Can you work these out from the model? Positions are in its coordinate system, mm. A direction names the side the tool comes from. Give positions to 0.01 mm unless a question says otherwise; leave off trailing zeros. Order: outer loops, then holes, each group sorted by start corner. A loop starts at its lowest first (then second) coordinate and runs counter-clockwise, first axis right, second up. Notation, with made-up numbers: M -15,33 L 40,33 A35 cw 40,70 Z; hole C 68.25,47 d5. An arc over 180 degrees is marked long. Write each question's results on one line, items separated by ' | '.
from build123d import *

# Parameters (mm, degrees)
SKETCH_1_R      = 1.5
SKETCH_1_W      = 87
SKETCH_1_H      = 57
EXTRUDE_2_DEPTH = 3
SKETCH_3_W      = 3
SKETCH_3_H      = 67
EXTRUDE_3_DEPTH = 2


with BuildPart() as part:
    # 草图1 → 凸台-拉伸2 (new body)
    with BuildSketch(Plane.XY):
        Polygon((-11.864484676, 21.655738596), (-19.864484676, 21.655738596), (-19.864484676, 10.655738596), (-19.864484676, -51.344261404), (-14.864484676, -51.344261404), (-11.864484676, -51.344261404), (98.135515324, -51.344261404), (98.135515324, -43.344261404), (98.135515324, 10.655738596), (98.135515324, 21.655738596), (-4.364484676, 21.655738596), (-6.864484676, 21.655738596), (-7.364484676, 21.655738596), align=None)
        with Locations((-11.864484676, -43.344261404)):
            Circle(SKETCH_1_R, mode=Mode.SUBTRACT)
        with Locations((90.135515324, -43.344261404)):
            Circle(SKETCH_1_R, mode=Mode.SUBTRACT)
        with Locations((-11.864484676, 13.655738596)):
            Circle(SKETCH_1_R, mode=Mode.SUBTRACT)
        with Locations((39.135515324, -14.844261404)):
            Rectangle(SKETCH_1_W, SKETCH_1_H, mode=Mode.SUBTRACT)
        with Locations((90.135515324, 13.655738596)):
            Circle(SKETCH_1_R, mode=Mode.SUBTRACT)
    extrude(amount=EXTRUDE_2_DEPTH)

    # 草图3 → 凸台-拉伸3 (add)
    with BuildSketch(Plane(origin=(0, 0, 0), x_dir=(-1, 0, 0), z_dir=(0, 0, -1))):
        with Locations((-96.635515324, -14.844261404)):
            Rectangle(SKETCH_3_W, SKETCH_3_H)
    extrude(amount=EXTRUDE_3_DEPTH)


solid = part.part
(1) We'd pull the mould along Y, two halves only. Please class faces 3 (the face through (-10.48, 13.08, 1.48)), 4 (the face through (40, 21.656, 1)), 5 (the face through (97, -14, -2)): +Y half, -Y half, draft (parallel to the pull), parting line (faces both ways), or undercut.
Data:
face 3: undercut | face 4: +Y half | face 5: draft
(2) Imagine slicing it at A-A, the plane x = 35. Write out the boundary of the cut face in (y, z).
Data:
outline: M -51.34,0 L -43.34,0 L -43.34,3 L -51.34,3 Z; M 13.66,0 L 21.66,0 L 21.66,3 L 13.66,3 Z
(3) I need wall thicknesses on L1, parallel to Y at x = 29, z = 1.1; L2, parallel to X at y = -2, z = 2.65; L3, parallel to Z at x = -5.5, y = -34.5. Which ranges of each line are inside material? Lowest first, please. Write a range as from..to.
Data:
L1: y = -51.34..-43.34, 13.66..21.66 | L2: x = -19.86..-4.36, 82.64..98.14 | L3: z = 0..3
(4) Will these pins go through, and if not, where does the flat tip stop? P1, Ø1, axis at x = 96, z = -1, coming from the +Y side; P2, Ø1.6, axis at x = 96.5, z = -1, coming from the -Y side.
Data:
P1: stops at y = 18.66 | P2: stops at y = -48.34
(5) Imagine slicing it at C-C, the plane z = 1.4. Write out the boundary of the cut face in (x, y), plus the area to 3 significant figures.
Data:
outline: M -19.86,-51.34 L 98.14,-51.34 L 98.14,21.66 L -19.86,21.66 Z; hole C -11.86,-43.34 d3; hole C -11.86,13.66 d3; hole M -4.36,-43.34 L 82.64,-43.34 L 82.64,13.66 L -4.36,13.66 Z; hole C 90.14,-43.34 d3; hole C 90.14,13.66 d3 | area: 3,630 mm2
(6) Imagine slicing it at B-B, the plane y = 1.5. Write out the boundary of the cut face in (x, z).
Data:
outline: M -19.86,0 L -4.36,0 L -4.36,3 L -19.86,3 Z; M 82.64,0 L 95.14,0 L 95.14,-2 L 98.14,-2 L 98.14,3 L 82.64,3 Z
(7) For faces 1 (the face through (38, -51.344, 1)), 2 (the face through (39, -43.344, 1)), which set-ups out of +Z, -Z, +X, -X, +Y, -Y let a thin tool reach every point of the face, with its end or its side?
Data:
face 1: +Z, -Z, +X, -X, -Y | face 2: +Z, -Z
(8) Imagine slicing it at D-D, the plane x = 85.5. Write out the boundary of the cut face in (y, z), plus the area to 3 significant figures.
Data:
outline: M -51.34,0 L 21.66,0 L 21.66,3 L -51.34,3 Z | area: 219 mm2
